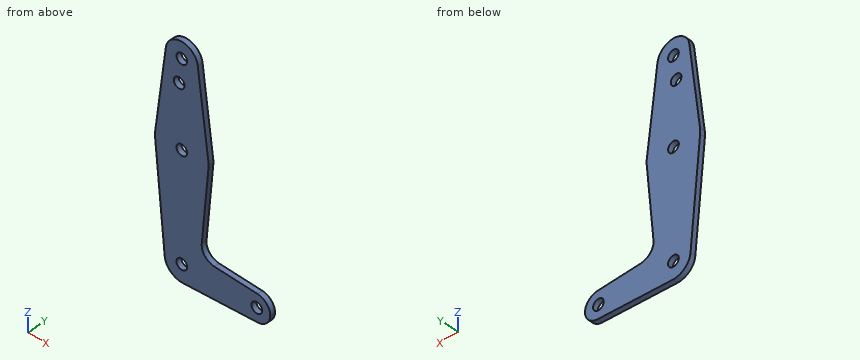
from build123d import *

# Parameters (mm, degrees)
F0_R     = 3.175
F1_DEPTH = 3.048


with BuildPart() as f1:
    # F0 (on Front) → F1 (new body)
    with BuildSketch(Plane.XZ):
        with BuildLine():
            ThreePointArc((0.508, -10.147292), (7.361619, -7.002297), (10.16, 0))
            ThreePointArc((10.16, 0), (-0.457665, 10.149687), (-10.118768, -0.9144))
            ThreePointArc((-10.118768, -0.9144), (-6.663579, -7.66957), (0.508, -10.147292))
        make_face()
        Circle(F0_R, mode=Mode.SUBTRACT)
        with BuildLine():
            ThreePointArc((-10.118768, -0.9144), (-0.457665, 10.149687), (10.16, 0))
            ThreePointArc((10.16, 0), (7.361619, -7.002297), (0.508, -10.147292))
            Line((0.508, -10.147292), (44.846875, -7.927572))
            ThreePointArc((44.846875, -7.927572), (36.5125, -0.001123), (44.844631, 7.927684))
            Line((44.844631, 7.927684), (19.337417, 9.197405))
            ThreePointArc((19.337417, 9.197405), (13.731979, 11.922673), (11.814743, 17.853291))
            Line((11.814743, 17.853291), (15.810576, 62.07125))
            ThreePointArc((15.810576, 62.07125), (0, 47.625), (-15.810576, 62.07125))
            Line((-15.810576, 62.07125), (-10.118768, -0.9144))
        make_face()
        with BuildLine():
            ThreePointArc((-15.750488, 65.484375), (-15.872541, 63.779432), (-15.810576, 62.07125))
            ThreePointArc((-15.810576, 62.07125), (0, 47.625), (15.810576, 62.07125))
            ThreePointArc((15.810576, 62.07125), (15.858886, 62.784899), (15.875, 63.5))
            ThreePointArc((15.875, 63.5), (15.843841, 64.494139), (15.750488, 65.484375))
            ThreePointArc((15.750488, 65.484375), (0, 79.375), (-15.750488, 65.484375))
        make_face()
        with Locations((0, 63.5)):
            Circle(F0_R, mode=Mode.SUBTRACT)
        with BuildLine():
            ThreePointArc((44.844631, 7.927684), (36.5125, -0.001123), (44.846875, -7.927572))
            ThreePointArc((44.846875, -7.927572), (50.201265, -5.470544), (52.3875, 0))
            ThreePointArc((52.3875, 0), (50.200491, 5.471358), (44.844631, 7.927684))
        make_face()
        with Locations((44.45, 0)):
            Circle(F0_R, mode=Mode.SUBTRACT)
        with BuildLine():
            Line((-9.450293, 115.490625), (-15.750488, 65.484375))
            ThreePointArc((-15.750488, 65.484375), (0, 79.375), (15.750488, 65.484375))
            Line((15.750488, 65.484375), (9.450293, 115.490625))
            ThreePointArc((9.450293, 115.490625), (9.506305, 114.896483), (9.525, 114.3))
            ThreePointArc((9.525, 114.3), (-0.596483, 104.793695), (-9.450293, 115.490625))
        make_face()
        with Locations((-1.5875, 100.0252)):
            Circle(F0_R, mode=Mode.SUBTRACT)
        with BuildLine():
            ThreePointArc((9.450293, 115.490625), (0, 123.825), (-9.450293, 115.490625))
            ThreePointArc((-9.450293, 115.490625), (-0.596483, 104.793695), (9.525, 114.3))
            ThreePointArc((9.525, 114.3), (9.506305, 114.896483), (9.450293, 115.490625))
        make_face()
        with Locations((0, 114.3)):
            Circle(F0_R, mode=Mode.SUBTRACT)
    extrude(amount=F1_DEPTH)


solid = f1.part
Work out the finished part from the listing and answer in its coordinate system (mm). Round coordinates to 2 decimals unless told otherwise and drop trailing zeros. Order: outer loops, then holes, each group sorted by start corner. A loop starts at its lowest first (then second) coordinate and runs counter-clockwise, first axis right, second up. Notation, with made-up numbers: M 53,-6 L 89,-6 A24 ccw 89,9 Z; hole C 42,-11 d5. An arc over 180 degrees is marked long. Put each result on its own line as item: value. Start each with the question number.
Q1. Straight lines are drawn through the part: L1, parallel to Z at x = 44.45, y = -2 (3 decimals); L2, parallel to X at y = -1.9, z = 1; L3, parallel to Z at x = 46.5, y = -1.35. For each, find the intervals that lie inside material, in ascending order. Write a range as [from, to].
Q2. Section A-A, the plane y = -2.2 is taken. Give the number of separate pieces and of enclosed holes in the cut face, and give its area (3 significant figures).
Q3. Section C-C, the plane z = 40 is taken. Write down the section's boundary in (x, y).
Q4. Section B-B, the plane x = 31.5 is taken. Write down the section's boundary in (y, z).
Findings below:
1. L1: z = [-7.947, -3.175], [3.175, 7.947]
1. L2: x = [-10.29, -3.01], [3.01, 41.44], [47.46, 52.32]
1. L3: z = [-7.67, -2.42], [2.42, 7.67]
2. separate pieces: 1
2. enclosed holes: 5
2. area: 3,840 mm^2
3. outline: M -13.82,-3.05 L 13.82,-3.05 L 13.82,0 L -13.82,0 Z
4. outline: M -3.05,-8.6 L 0,-8.6 L 0,8.59 L -3.05,8.59 Z
